Print and shaded views of the part. All mm, measured from the part's lowest x, y and z. A direction names the side the tool comes from. Round coordinates to 2 decimals unless told otherwise and drop trailing zeros. Loops run counter-clockwise (first coordinate to the right, second up) from the corner with the lowest first, then second, coordinate; pieces in that order, holes last. Notation, with made-up numbers: (79.25, 3.5) - (128.25, 3.5) arc R13 cw to (128.25, 11.5) - close; hole circle Ø7 at (-29, 86.5). An arc over 180 degrees is marked (long way). Use one line per item in the form item = value. Start each with the question number.
Q1. Saw through at D-D (z = 229). Give the cut face in (x, y).
Q2. Saw through at C-C (y = 14). Give the cut face in (x, z).
Q3. Saw through at B-B (x = 80). Give the cut face in (y, z).
Q4. 3-axis set-ups, long thin cutter, end or side, ignore diameter. For the marked faces 1, 2 and 3: which of +Z, -Z, +X, -X, +Y, -Y reach the whole face in a straight line?
Q5. Pin check, flat tips, straight feed: pin 1 (22 mm diameter, centred on x = 58.5, z = 13, fed in from +Y); pin 2 (1.5 mm diameter, centred on x = 95.5, y = 106, fed in from -Z); pin 3 (2 mm diameter, centred on x = 76, z = 196.5, fed in from -Y); pin 4 (6 mm diameter, centred on x = 49, z = 13.5, fed in from -Y). Stop position of each tip, or through.
Q6. Saw through at A-A (y = 115.5). Give the cut face in (x, z).
Q7. Drill centre lines: line 1 (X direction, y = 14, z = 11.5); line 2 (Y direction, x = 31.5, z = 144.5); line 3 (Z direction, x = 81, y = 62). Where is each one in solid material? Low to high.
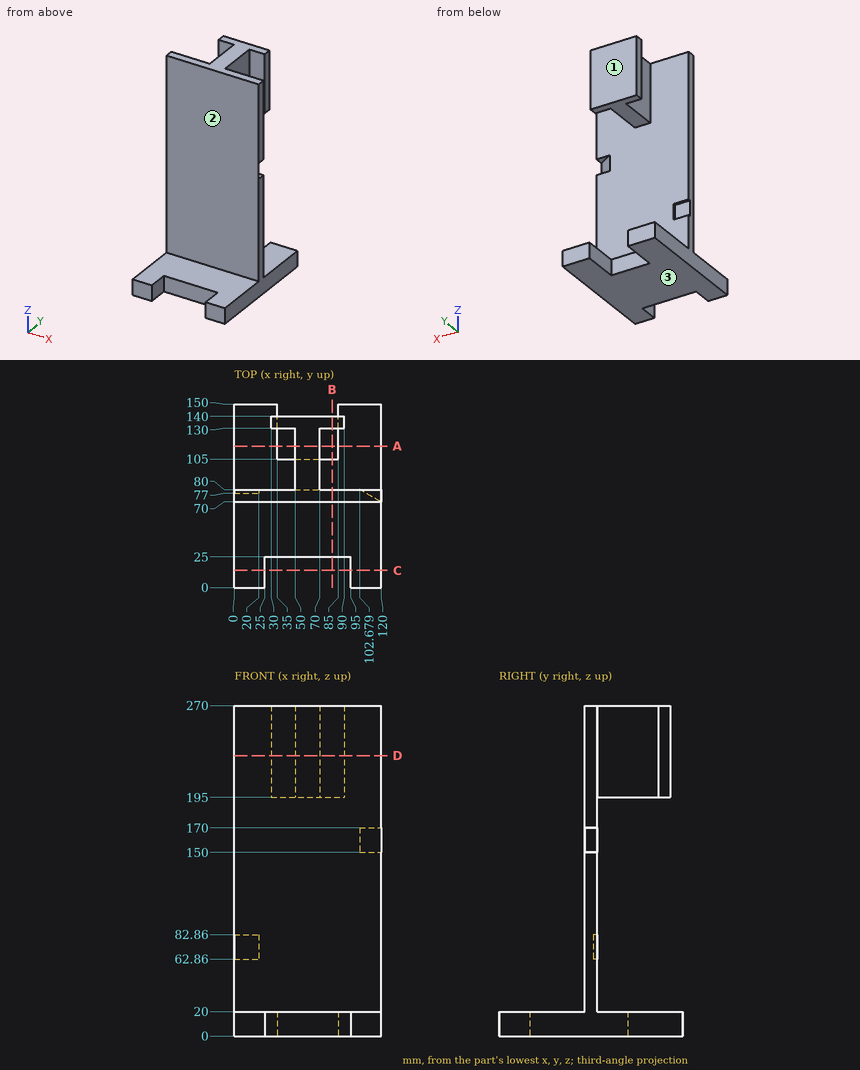
Report:
q1.outline = (0, 70) - (120, 70) - (120, 80) - (70, 80) - (70, 130) - (90, 130) - (90, 140) - (30, 140) - (30, 130) - (50, 130) - (50, 80) - (0, 80) - close
q2.outline = (0, 0) - (25, 0) - (25, 20) - (0, 20) - close; (95, 0) - (120, 0) - (120, 20) - (95, 20) - close
q3.outline = (25, 0) - (105, 0) - (105, 20) - (80, 20) - (80, 270) - (70, 270) - (70, 20) - (25, 20) - close; (130, 195) - (140, 195) - (140, 270) - (130, 270) - close
q4.face_1 = +Z, +X, -X, +Y
q4.face_2 = +Z, +X, -X, -Y
q4.face_3 = -Z, +X, -X, +Y, -Y
q5.pin_1 = 105
q5.pin_2 = 0
q5.pin_3 = 70
q5.pin_4 = 25
q6.outline = (0, 0) - (35, 0) - (35, 20) - (0, 20) - close; (50, 195) - (70, 195) - (70, 270) - (50, 270) - close; (85, 0) - (120, 0) - (120, 20) - (85, 20) - close
q7.line_1 = 0 to 25, 95 to 120
q7.line_2 = 70 to 80
q7.line_3 = 0 to 20
